Input: part model. Units: mm. Frame: model coordinates. Face numbers are marked on the shaded views. A direction names the side the tool comes from. Coordinates: 2 decimals unless noted, no trailing zeros. Order: outer loops, then holes, each group sorted by start corner. A loop starts at its lowest first (then second) coordinate and runs counter-clockwise, first axis right, second up. Notation, with made-up numbers: M 44,46.25 L 92,46.25 A13 cw 92,62.25 Z; hole C -36,-19 d3. An arc over 180 degrees is marked long. One line per item, written item: value.
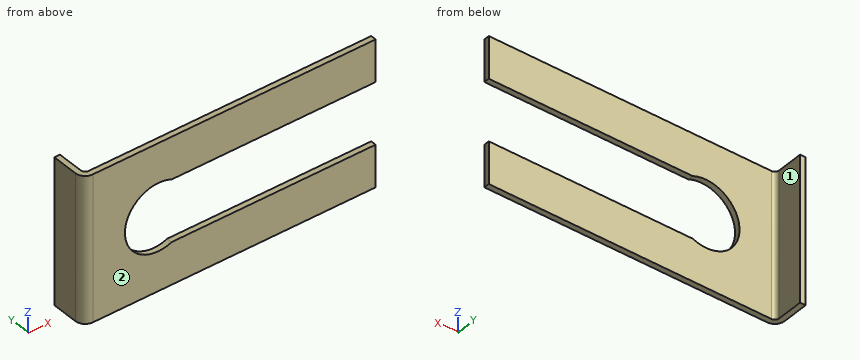
```python
from build123d import *

# Parameters (mm, degrees)
T_LE_DE_BASE_PLI_E1_DEPTH             = 1
T_LE_PLI_E_SUR_AR_TE1_STRIP_W         = 5.4732
T_LE_PLI_E_SUR_AR_TE1_STRIP_H         = 1
T_LE_PLI_E_SUR_AR_TE1_STRIP_CUT_DEPTH = 26
T_LE_PLI_E_SUR_AR_TE1_DEPTH           = 26


# Sheet-metal steps are written as plain solids
with BuildPart() as part:
    # Esquisse1 → Tôle de base pliée1 (new body)
    with BuildSketch(Plane(origin=(0, 0, 0), x_dir=(1, 0, 0), z_dir=(0, 1, 0))):
        with BuildLine():
            Line((-26.25, -13), (26.25, -13))
            Line((26.25, -13), (26.25, -5.5))
            Line((26.25, -5.5), (-10.352084238, -5.5))
            ThreePointArc((-10.352084238, -5.5), (-18.75, 0), (-10.352084238, 5.5))
            Line((-10.352084238, 5.5), (26.25, 5.5))
            Line((26.25, 5.5), (26.25, 13))
            Line((26.25, 13), (-26.25, 13))
            Line((-26.25, 13), (-26.25, -13))
        make_face()
    extrude(amount=-T_LE_DE_BASE_PLI_E1_DEPTH)

    # Tôle pliée sur arête1 strip (across the edge) → Tôle pliée sur arête1 strip cut (cut)
    with BuildSketch(Plane(origin=(-26.25, 0, -13), x_dir=(1, 0, 0), z_dir=(0, 0, 1))):
        with Locations((-1, -0.5)):
            Rectangle(T_LE_PLI_E_SUR_AR_TE1_STRIP_W, T_LE_PLI_E_SUR_AR_TE1_STRIP_H)
    extrude(amount=T_LE_PLI_E_SUR_AR_TE1_STRIP_CUT_DEPTH, mode=Mode.SUBTRACT)

    # Tôle pliée sur arête1 section (across the edge) → Tôle pliée sur arête1 (add)
    with BuildSketch(Plane(origin=(-26.25, 0, -13), x_dir=(1, 0, 0), z_dir=(0, 0, 1))):
        with BuildLine():
            Line((0, 0.7366), (0, 5.5))
            Line((0, 5.5), (1, 5.5))
            Line((1, 5.5), (1, 0.7366))
            ThreePointArc((1, 0.7366), (1.215745145, 0.215745145), (1.7366, 0))
            Line((1.7366, 0), (1.7366, -1))
            ThreePointArc((1.7366, -1), (0.508638364, -0.491361636), (0, 0.7366))
        make_face()
    extrude(amount=T_LE_PLI_E_SUR_AR_TE1_DEPTH)


solid = part.part
```
(1) Cut plane B-B on x = 6.5. Output: boundary loops of the cut face in (y, z).
Data:
outline: M -1,-13 L 0,-13 L 0,-5.5 L -1,-5.5 Z; M -1,5.5 L 0,5.5 L 0,13 L -1,13 Z
(2) Access query for the marked faces 1 and 2. Directions: +Z, -Z, +X, -X, +Y, -Y. A direction counts if a zero-diameter tool reaches every point of the face in a straight line with its end or side. Return the directions, or none.
Data:
face 1: +Z, -Z, +X, +Y
face 2: +Z, -Z, +X, -X, -Y
(3) Cut plane A-A on x = -12.75. Output: boundary loops of the cut face in (y, z), plus the area to 3 significant figures.
Data:
outline: M -1,-13 L 0,-13 L 0,-6 L -1,-6 Z; M -1,6 L 0,6 L 0,13 L -1,13 Z
area: 14.0 mm2
(4) Ray query, line 1 (Z direction, x = 11.5, y = -0.5); line 2 (Z direction, x = -12.75, y = -0.6); line 3 (Y direction, x = -14.5, z = 12). Return the intervals inside material, ascending. Write a range as from..to.
Data:
line 1: z = -13..-5.5, 5.5..13
line 2: z = -13..-6, 6..13
line 3: y = -1..0
(5) Cut plane D-D on y = 3. Output: boundary loops of the cut face in (x, z), plus the area to 3 significant figures.
Data:
outline: M -26.25,-13 L -25.25,-13 L -25.25,13 L -26.25,13 Z
area: 26.0 mm2
(6) Cut plane C-C on z = 9. Output: boundary loops of the cut face in (x, y).
Data:
outline: M -26.25,0.74 A1.74 ccw -24.51,-1 L 26.25,-1 L 26.25,0 L -24.51,0 A0.74 cw -25.25,0.74 L -25.25,5.5 L -26.25,5.5 Z
(7) First-contact query: pin 1 (2.5 mm diameter, centred on y = 3, z = -5.5, fed in from +X); pin 2 (1.5 mm diameter, centred on y = 0.5, z = -2, fed in from +X); pin 3 (4 mm diameter, centred on x = 1.5, z = -5.5, fed in from +Y). Flat tips, straight axial feed; report the tip coordinate or a pass-through.
Data:
pin 1: stops at x = -25.25
pin 2: stops at x = -18.18
pin 3: stops at y = 0
